```python
from build123d import *

# Parameters (mm, degrees)
CROQUIS1_W              = 100
CROQUIS1_H              = 127.304752994
SALIENTE_EXTRUIR1_DEPTH = 3
CROQUIS2_W              = 3
CROQUIS2_H              = 31.14357053
SALIENTE_EXTRUIR2_DEPTH = 60
CROQUIS3_R              = 2.5
SALIENTE_EXTRUIR3_DEPTH = 10


with BuildPart() as part:
    # Croquis1 → Saliente-Extruir1 (new body)
    with BuildSketch(Plane(origin=(0, 0, 0), x_dir=(1, 0, 0), z_dir=(0, 1, 0))):
        Rectangle(CROQUIS1_W, CROQUIS1_H)
    extrude(amount=SALIENTE_EXTRUIR1_DEPTH)

    # Croquis2 → Saliente-Extruir2 (add)
    with BuildSketch(Plane.XZ):
        with Locations((33.110839978, -1.924439839)):
            Rectangle(CROQUIS2_W, CROQUIS2_H)
    extrude(amount=SALIENTE_EXTRUIR2_DEPTH)

    # Croquis3 → Saliente-Extruir3 (add)
    with BuildSketch(Plane(origin=(0, 3, 0), x_dir=(1, 0, 0), z_dir=(0, 1, 0))):
        with Locations(Location((11.26131509, 46.378735673, 0), (0, 0, 270))):
            Circle(CROQUIS3_R)
        with Locations(Location((11.26131509, 17.087366944, 0), (0, 0, 270))):
            Circle(CROQUIS3_R)
        with Locations(Location((-33.233745319, 17.087366944, 0), (0, 0, 270))):
            Circle(CROQUIS3_R)
        with Locations(Location((-33.233745319, 46.378735673, 0), (0, 0, 270))):
            Circle(CROQUIS3_R)
    extrude(amount=SALIENTE_EXTRUIR3_DEPTH)


solid = part.part
```
Input: part model. Units: mm. Frame: model coordinates. A direction names the side the tool comes from. Coordinates: 2 decimals unless noted, no trailing zeros. Write each loop counter-clockwise with the first axis right and the second up, starting at its lowest first coordinate (ties: lowest second). Pieces come first, ordered by that corner, then holes.
1) Section B-B on y = -9. Output: boundary loops of the cut face in (x, z).
2) Mould query, pull axis Z, two halves, no side actions, for faces 1 (the flat face through (-1, 1, -63.652)), 2 (the flat face through (-33, 13, -17)), 3 (the cylindrical face through (11.371, 7.93, -19.585)). Classes: pulls with the +Z half, pulls with the -Z half, needs draft (parallel to the pull), parting line crosses it, or undercut.
3) Material intervals for line 1 along Y through (x, z) = (-23.5, 16); line 2 along X through (y, z) = (-36.5, -5.5); line 3 along Z through (x, y) = (32, -34), sorted ascending.
4) Section C-C on x = 38. Output: boundary loops of the cut face in (y, z), and give its area (3 significant figures).
5) Set-up query: faces 4 (the flat face through (33, -30, -17.496)), 5 (the flat face through (33, -30, 13.647)), 6 (the flat face through (31.611, -30, -2)), 7 (the flat face through (34.611, -30, -2)). Return all of +Z, -Z, +X, -X, +Y, -Y with unobstructed straight access to the full face (end or side cutting, diameter ignored); none if empty.
6) Pin query (flat end, axial travel): pin 1 Ø15.5 at (y, z) = (-16, -6) entering from +X; pin 2 Ø2.5 at (x, y) = (33.5, -15.5) entering from +Z; pin 3 Ø3 at (x, z) = (-19.5, 43.5) entering from -Y. Return the tip coordinate at first contact, or that it passes through.
7) Section A-A on z = -2. Output: boundary loops of the cut face in (x, y), and give its area (3 significant figures).
8) Section D-D on y = 6.5. Output: boundary loops of the cut face in (x, z).
Check result:
1. outline: (31.61, -17.5) - (34.61, -17.5) - (34.61, 13.65) - (31.61, 13.65) - close
2. face 1: pulls with the -Z half
2. face 2: needs draft
2. face 3: undercut
3. line 1: y = 0 to 3
3. line 2: x = 31.61 to 34.61
3. line 3: z = -17.5 to 13.65
4. outline: (0, -63.65) - (3, -63.65) - (3, 63.65) - (0, 63.65) - close
4. area: 382 mm2
5. face 4: -Z, +X, -X, -Y
5. face 5: +Z, +X, -X, -Y
5. face 6: +Z, -Z, -X, -Y
5. face 7: +Z, -Z, +X, -Y
6. pin 1: stops at x = 34.61
6. pin 2: stops at z = 13.65
6. pin 3: stops at y = 0
7. outline: (-50, 0) - (31.61, 0) - (31.61, -60) - (34.61, -60) - (34.61, 0) - (50, 0) - (50, 3) - (-50, 3) - close
7. area: 480 mm2
8. outline: circle Ø5 at (-33.23, -46.38); circle Ø5 at (-33.23, -17.09); circle Ø5 at (11.26, -46.38); circle Ø5 at (11.26, -17.09)
